from build123d import *

# Parameters (mm, degrees)
SKETCH21_R           = 1.7
SKETCH21_W           = 26.12
SKETCH21_H           = 7.66
BOSS_EXTRUDE18_DEPTH = 6


with BuildPart() as part:
    # Sketch21 → Boss-Extrude18 (new body)
    with BuildSketch(Plane(origin=(0, 0, 0), x_dir=(1, 0, 0), z_dir=(0, 1, 0))):
        Polygon((-0.002759086, 59.199662961), (-16.062759086, 59.199662961), (-16.062759086, 16.199662961), (-59.062759086, 16.199662961), (-59.062759086, 0.139662961), (-59.062759086, -15.920337039), (-16.062759086, -15.920337039), (-16.062759086, -58.920337039), (-0.002759086, -58.920337039), (16.057240914, -58.920337039), (16.057240914, -15.920337039), (59.057240914, -15.920337039), (59.057240914, 0.139662961), (59.057240914, 16.199662961), (16.057240914, 16.199662961), (16.057240914, 59.199662961), align=None)
        with Locations(Location((-12.56, 6.44, 0), (0, 0, 270))):
            Circle(SKETCH21_R, mode=Mode.SUBTRACT)
        with Locations(Location((12.56, 6.44, 0), (0, 0, 270))):
            Circle(SKETCH21_R, mode=Mode.SUBTRACT)
        with Locations((0, -3.83)):
            Rectangle(SKETCH21_W, SKETCH21_H, mode=Mode.SUBTRACT)
    extrude(amount=BOSS_EXTRUDE18_DEPTH)


solid = part.part
Check sheet for the modelled part. Datum: model origin and axes. Units: mm. A direction names the side the tool comes from. Give positions to 0.01 mm unless a question says otherwise; leave off trailing zeros. Write each loop counter-clockwise with the first axis right and the second up, starting at its lowest first coordinate (ties: lowest second). Pieces come first, ordered by that corner, then holes. Notation, with made-up numbers: M -22,-13.5 L -15,-13.5 A35 ccw -15,25.5 Z; hole C 0,16 d8. An arc over 180 degrees is marked long. Use one line per item in the form item = value.
(1) Material ranges on line 1 along X through (y, z) = (2.15, -6.44); line 2 along X through (y, z) = (2.85, -51); line 3 along Z through (x, y) = (4, 1.5), recorded low to high.
Answer block:
line_1 = -59.06 to -14.26, -10.86 to 10.86, 14.26 to 59.06
line_2 = -16.06 to 16.06
line_3 = -59.2 to 0, 7.66 to 58.92
(2) Section check B-B on y = 2.85. Record the boundary of the cut face in (x, z).
Answer block:
outline = M -59.06,-16.2 L -16.06,-16.2 L -16.06,-59.2 L 16.06,-59.2 L 16.06,-16.2 L 59.06,-16.2 L 59.06,15.92 L 16.06,15.92 L 16.06,58.92 L -16.06,58.92 L -16.06,15.92 L -59.06,15.92 Z; hole C -12.56,-6.44 d3.4; hole M -13.06,0 L 13.06,0 L 13.06,7.66 L -13.06,7.66 Z; hole C 12.56,-6.44 d3.4
(3) Section check A-A on z = 6. Record the boundary of the cut face in (x, y).
Answer block:
outline = M -59.06,0 L -13.06,0 L -13.06,6 L -59.06,6 Z; M 13.06,0 L 59.06,0 L 59.06,6 L 13.06,6 Z
(4) Section check C-C on z = -6.44. Record the boundary of the cut face in (x, y).
Answer block:
outline = M -59.06,0 L -14.26,0 L -14.26,6 L -59.06,6 Z; M -10.86,0 L 10.86,0 L 10.86,6 L -10.86,6 Z; M 14.26,0 L 59.06,0 L 59.06,6 L 14.26,6 Z
(5) Tool access check on faces 5 (the flat face through (-37, 3, -16.2)), 6 (the flat face through (-16.063, 3, 37)), 7 (the flat face through (37, 3, 15.92)), 8 (the flat face through (16.057, 3, -37)), 9 (the flat face through (-13.06, 3, 4)). Record the directions out of +Z, -Z, +X, -X, +Y, -Y that give a thin tool (end or side, any length) a straight path to the whole face; none if there is none.
Answer block:
face_5 = -Z, -X, +Y, -Y
face_6 = +Z, -X, +Y, -Y
face_7 = +Z, +X, +Y, -Y
face_8 = -Z, +X, +Y, -Y
face_9 = +Y, -Y
(6) Draft check along Z on faces 1 (the flat face through (16.057, 3, 38)), 2 (the cylindrical face through (14.246, 2.958, -6.661)), 3 (the flat face through (0, 3, -59.2)), 4 (the flat face through (0, 3, 7.66)). Enter one of: pulls with the +Z half, pulls with the -Z half, needs draft (parallel to the pull), parting line crosses it, or undercut.
Answer block:
face_1 = needs draft
face_2 = undercut
face_3 = pulls with the -Z half
face_4 = undercut
(7) Section check D-D on x = -48. Record the boundary of the cut face in (y, z).
Answer block:
outline = M 0,-16.2 L 6,-16.2 L 6,15.92 L 0,15.92 Z
(8) Depth check by flat-ended pin: P1, Ø1.8, axis at y = 2.5, z = 41, coming from the +X side; P2, Ø1, axis at x = 26, y = 5, coming from the +Z side; P3, Ø1.8, axis at x = 46.5, y = 3, coming from the -Z side. Enter the tip coordinate at first touch or a pass-through.
Answer block:
P1 = 16.06
P2 = 15.92
P3 = -16.2
